Source: three-view drawing plus pictorial views. Frame: mm from the lowest corner of the part. Round coordinates to 2 decimals unless told otherwise and drop trailing zeros. Loops run counter-clockwise (first coordinate to the right, second up) from the corner with the lowest first, then second, coordinate; pieces in that order, holes last. Notation, with made-up numbers: M -15.75,-4.5 L 14.25,-4.5 A10 cw 14.25,11.5 Z; hole C 44.5,-19.5 d5. An arc over 180 degrees is marked long. Answer as a JSON object with one key per item and string values.
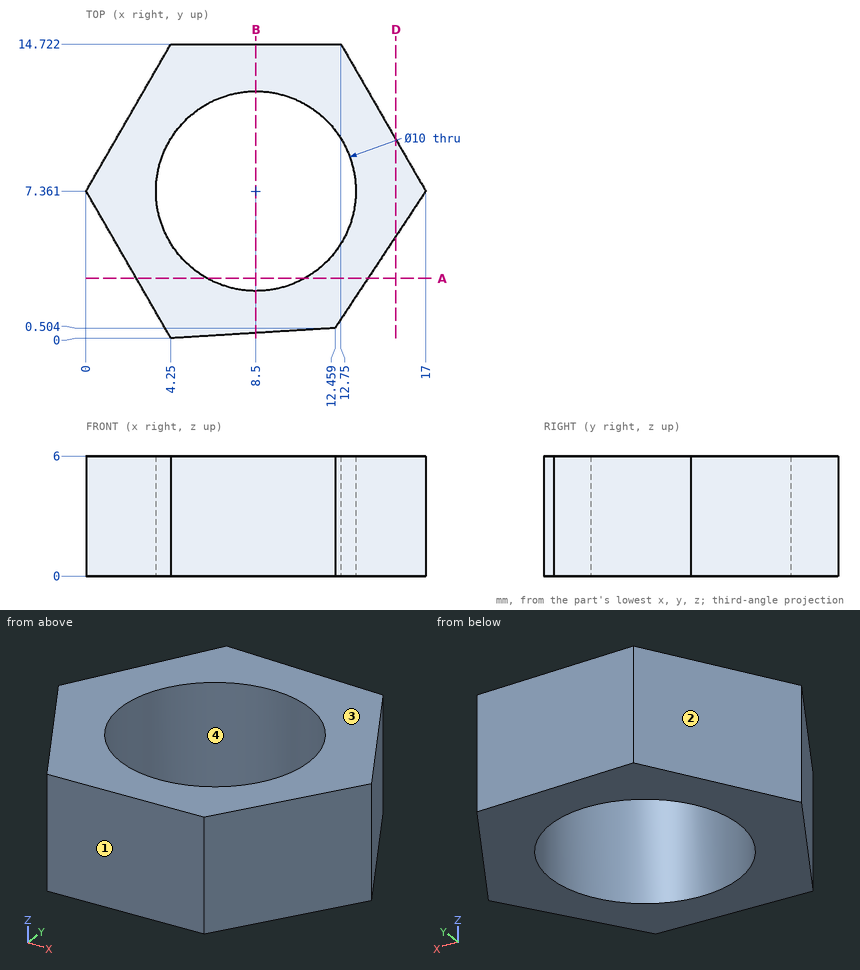
1) Line query: probe 1 along X at (y, z) = (8, 4.45); probe 2 along X at (y, z) = (10.5, 1.6); probe 3 along Y at (x, z) = (9, 4.05). Output: solid intervals per line, ascending.
Geometry results:
{"probe 1": "0.37 to 3.54, 13.46 to 16.63", "probe 2": "1.81 to 4.61, 12.39 to 15.19", "probe 3": "0.29 to 2.39, 12.34 to 14.72"}
2) Cut plane A-A on y = 3. Return the cut outline in (x, z) (1 decimal), and give its area (3 significant figures).
Geometry results:
{"outline": "M 2.5,0 L 6.1,0 L 6.1,6 L 2.5,6 Z; M 10.9,0 L 14.1,0 L 14.1,6 L 10.9,6 Z", "area": "40.2 mm2"}
3) First-contact query: pin 1 (2 mm diameter, centred on y = 9.5, z = 4.5, fed in from +X). Flat tip, straight axial feed; report the tip coordinate or a pass-through.
Geometry results:
{"pin 1": "x = 16.34"}
4) Cut plane D-D on x = 15.5. Return the cut outline in (y, z).
Geometry results:
{"outline": "M 5.1,0 L 9.96,0 L 9.96,6 L 5.1,6 Z"}
5) Cut plane B-B on x = 8.5. Return the cut outline in (y, z).
Geometry results:
{"outline": "M 0.26,0 L 2.36,0 L 2.36,6 L 0.26,6 Z; M 12.36,0 L 14.72,0 L 14.72,6 L 12.36,6 Z"}
6) Pull-direction query (X, two-part tool) for the marked faces 1, 2, 3 and 4; classes: +X half, -X half, draft (parallel to the pull), parting line (faces both ways), or undercut.
Geometry results:
{"face 1": "+X half", "face 2": "-X half", "face 3": "draft", "face 4": "undercut"}
